For this review, take the finished solid that the model builds, in its own axes (mm). A direction names the side the tool comes from. Coordinates: 2 decimals unless noted, no trailing zeros. Order: outer loops, then holes, each group sorted by start corner. A loop starts at its lowest first (then second) coordinate and runs counter-clockwise, first axis right, second up. Notation, with made-up numbers: (-22.5, 89.25) -> (17.5, 89.25) arc R25 ccw to (17.5, 127.25) -> close; hole circle Ø2 at (-10, 61.25). An arc over 180 degrees is marked (long way). Return JSON: item names as keys, results as strings. Group by question number.
Item 1: Take a section at A-A (y = -30). Write out the cut boundary in (x, z).
Item 2: Machinability: for faces 5 (the flat face through (-35.4, 33, 12)), 6 (the flat face through (-20, 5, 12)), 7 (the flat face through (-18, -17, 3)), 8 (the flat face through (-30.4, -17, 1)), 9 (the flat face through (-5, -17, 1)), which of the approach directions +Z, -Z, +X, -X, +Y, -Y give a long, thin tool a straight path to every point of the face, cutting with its end or side? Answer none if there is none.
Item 3: Take a section at C-C (y = -9). Write out the cut boundary in (x, z), then the cut area to 3 significant figures.
Item 4: Take a section at D-D (z = 9.75). Write out the cut boundary in (x, y), then the cut area to 3 significant figures.
Item 5: Take a section at B-B (x = -32.5). Write out the cut boundary in (y, z), then the cut area to 3 significant figures.
Item 6: For line 1 along Y through (x, z) = (-34, 14.5); line 2 along Z through (x, y) = (-26, -6); line 3 along Y through (x, z) = (-25, 21.25), list the stretches that pass through material, from the lowest coordinate up.
Item 7: Draft analysis for pull direction X (two halves, no side actions). For faces 1 (the cylindrical face through (-23.552, -28.356, 1.479)), 2 (the flat face through (0, 17, 12)), 3 (the flat face through (-18, 1, 24)), 4 (the cylindrical face through (-11.054, -28.067, 1.479)), state which applies: +X half, -X half, draft (parallel to the pull), parting line (faces both ways), or undercut.
Item 8: Insertion check: pin 1 (5 mm diameter, centred on x = -24.6, y = -30, fed in from +Z); pin 2 (1 mm diameter, centred on x = -32, z = 13.5, fed in from -Y); pin 3 (1.5 mm diameter, centred on y = -14.5, z = 1, fed in from -X); pin 4 (3.5 mm diameter, centred on x = -10.8, y = -30, fed in from +Z). Each pin has a flat end and moves straight along its axis. Give the tip position at first contact, or say it passes through.
```python
from build123d import *

# Parameters (mm, degrees)
SKETCH1_R           = 1.95
SKETCH1_W           = 25.4
SKETCH1_H           = 25.4
BOSS_EXTRUDE1_DEPTH = 24
SKETCH3_W           = 18
SKETCH3_H           = 34
CUT_EXTRUDE1_DEPTH  = 56.518645517
CUT_EXTRUDE2_REACH  = 83.52
SKETCH4_R           = 2.75
SKETCH5_W           = 5
SKETCH5_H           = 25.4
CUT_EXTRUDE3_DEPTH  = 56.518645517


with BuildPart() as part:
    # Sketch1 → Boss-Extrude1 (new body)
    with BuildSketch(Plane.XY):
        Polygon((0, 0), (0, 35.4), (-35.4, 35.4), (-35.4, 0), (-30.4, 0), (-30.4, -34), (-5, -34), (-5, 0), align=None)
        with Locations((-24.6, -30)):
            Circle(SKETCH1_R, mode=Mode.SUBTRACT)
        with Locations((-10.8, -30)):
            Circle(SKETCH1_R, mode=Mode.SUBTRACT)
        with Locations((-17.7, 17.7)):
            Rectangle(SKETCH1_W, SKETCH1_H, mode=Mode.SUBTRACT)
    extrude(amount=BOSS_EXTRUDE1_DEPTH)

    # Sketch3 → Cut-Extrude1 (cut, through all)
    with BuildSketch(Plane.ZY.offset(35.4)):
        with Locations((12, -17)):
            Rectangle(SKETCH3_W, SKETCH3_H)
    extrude(amount=-CUT_EXTRUDE1_DEPTH, mode=Mode.SUBTRACT)

    # Sketch4 → Cut-Extrude2 (cut, up to next)
    with BuildSketch(Plane(origin=(0, 35.4, 0), x_dir=(1, 0, 0), z_dir=(0, 1, 0)), mode=Mode.PRIVATE) as cut_extrude2_sk1:
        with Locations(Location((-17.7, -6, 0), (0, 0, 180))):
            Circle(SKETCH4_R)
    cut_extrude2_tool1 = extrude(cut_extrude2_sk1.sketch, amount=-CUT_EXTRUDE2_REACH, mode=Mode.PRIVATE) & part.part
    # Sketch4 → Cut-Extrude2 (cut, up to next)
    with BuildSketch(Plane(origin=(0, 35.4, 0), x_dir=(1, 0, 0), z_dir=(0, 1, 0)), mode=Mode.PRIVATE) as cut_extrude2_sk2:
        with Locations(Location((-17.7, -18, 0), (0, 0, 180))):
            Circle(SKETCH4_R)
    cut_extrude2_tool2 = extrude(cut_extrude2_sk2.sketch, amount=-CUT_EXTRUDE2_REACH, mode=Mode.PRIVATE) & part.part
    add(cut_extrude2_tool1.solids().sort_by_distance((-17.7, 35.4, 6))[0], mode=Mode.SUBTRACT)
    add(cut_extrude2_tool2.solids().sort_by_distance((-17.7, 35.4, 18))[0], mode=Mode.SUBTRACT)

    # Sketch5 → Cut-Extrude3 (cut, through all)
    with BuildSketch(Plane(origin=(0, 0, 0), x_dir=(-1, 0, 0), z_dir=(0, 0, -1))):
        with Locations((32.9, 17.7)):
            Rectangle(SKETCH5_W, SKETCH5_H)
    extrude(amount=-CUT_EXTRUDE3_DEPTH, mode=Mode.SUBTRACT)


solid = part.part
```
Findings below:
{
 "1": {"outline": "(-30.4, 0) -> (-26.55, 0) -> (-26.55, 3) -> (-30.4, 3) -> close; (-30.4, 21) -> (-26.55, 21) -> (-26.55, 24) -> (-30.4, 24) -> close; (-22.65, 0) -> (-12.75, 0) -> (-12.75, 3) -> (-22.65, 3) -> close; (-22.65, 21) -> (-12.75, 21) -> (-12.75, 24) -> (-22.65, 24) -> close; (-8.85, 0) -> (-5, 0) -> (-5, 3) -> (-8.85, 3) -> close; (-8.85, 21) -> (-5, 21) -> (-5, 24) -> (-8.85, 24) -> close"},
 "2": {"face 5": "+Z, -Z, -X, +Y, -Y", "face 6": "+Z, -Z, -X", "face 7": "+X, -X, -Y", "face 8": "+Z, -Z, -X, -Y", "face 9": "+Z, -Z, +X, -Y"},
 "3": {"outline": "(-30.4, 0) -> (-5, 0) -> (-5, 3) -> (-30.4, 3) -> close; (-30.4, 21) -> (-5, 21) -> (-5, 24) -> (-30.4, 24) -> close", "area": "152 mm2"},
 "4": {"outline": "(-35.4, 0) -> (0, 0) -> (0, 35.4) -> (-35.4, 35.4) -> (-35.4, 30.4) -> (-5, 30.4) -> (-5, 5) -> (-35.4, 5) -> close", "area": "481 mm2"},
 "5": {"outline": "(0, 0) -> (5, 0) -> (5, 24) -> (0, 24) -> close; (30.4, 0) -> (35.4, 0) -> (35.4, 24) -> (30.4, 24) -> close", "area": "240 mm2"},
 "6": {"line 1": "y = 0 to 5, 30.4 to 35.4", "line 2": "z = 0 to 3, 21 to 24", "line 3": "y = -34 to -31.91, -28.09 to 5, 30.4 to 35.4"},
 "7": {"face 1": "undercut", "face 2": "+X half", "face 3": "draft", "face 4": "undercut"},
 "8": {"pin 1": "stops at z = 24", "pin 2": "stops at y = 0", "pin 3": "stops at x = -30.4", "pin 4": "passes through"}
}
